Build history of the part. All positions in model axes, mm. A direction names the side the tool comes from. Round coordinates to 2 decimals unless told otherwise and drop trailing zeros. Loops run counter-clockwise (first coordinate to the right, second up) from the corner with the lowest first, then second, coordinate; pieces in that order, holes last. Notation, with made-up numbers: (-34, 4) - (-7, 4) arc R22 cw to (-7, 17) - close; hole circle Ø9 at (-27.5, -17.75). An arc over 180 degrees is marked (long way). Put each result on its own line as item: value. Start each with the question number.
from build123d import *

# Parameters (mm, degrees)
F0_W     = 50.8
F0_H     = 50.8
F1_DEPTH = 7.62
F2_T     = -1.27
F3_W     = 1.27
F3_H     = 6.604
F3_W_2   = 7.62
F3_H_2   = 1.27
F4_DEPTH = 6.35
F5_R     = 1.27
F6_DEPTH = 25.4


with BuildPart() as f1:
    # F0 (on Top) → F1 (new body)
    with BuildSketch(Plane.XY):
        with Locations((25.4, 25.4)):
            Rectangle(F0_W, F0_H)
    extrude(amount=F1_DEPTH)

    # F2
    f2_openings = [f1.faces().sort_by_distance(p)[0] for p in [
        (25.4, 25.4, 7.62),
    ]]
    offset(amount=F2_T, openings=f2_openings)

    # F3 (on face) → F4 (join)
    with BuildSketch(Plane.XY.offset(1.27)):
        Polygon((6.35, 42.545278), (6.35, 1.27), (7.62, 1.27), (7.62, 41.275278), (7.62, 42.545278), align=None)
        Polygon((7.62, 42.545278), (7.62, 41.275278), (39.37, 41.275278), (40.64, 41.275278), (40.64, 42.545278), align=None)
        with Locations((40.005, 37.973278)):
            Rectangle(F3_W, F3_H)
        with Locations((24.184101, 35.050092)):
            Rectangle(F3_W_2, F3_H_2)
    extrude(amount=F4_DEPTH)

    # F5 (on face) → F6 (cut)
    with BuildSketch(Plane.XY.offset(1.27)):
        with Locations((3.990767, 5.742811)):
            Circle(F5_R)
        with Locations((3.796095, 10.80427)):
            Circle(F5_R)
    extrude(amount=-F6_DEPTH, mode=Mode.SUBTRACT)


solid = f1.part
Item 1: Slice it at C-C (y = 38). Give the cut face in (x, z), plus the area to 3 significant figures.
Item 2: Two-plate mould, pull along Y, no slides. Class faces 1 (the flat face through (28, 1.27, 4)), 2 (the flat face through (0, 25, 4)), 3 (the flat face through (25, 0, 4)): pulls with the +Y half, pulls with the -Y half, needs draft (parallel to the pull), parting line crosses it, or undercut.
Item 3: Slice it at D-D (x = 44). Give the cut face in (y, z), plus the area to 3 significant figures.
Item 4: Slice it at A-A (z = 7). Give the cut face in (x, y).
Item 5: Drill centre lines: probe 1 along X at (y, z) = (27, 3); probe 2 along Y at (x, z) = (19, 5.75); probe 3 along X at (y, z) = (38.5, 6.75). Where is each one in solid material? Low to high. Write a range as [from, to].
Item 6: Which spindle directions (+Z, -Z, +X, -X, +Y, -Y) get a long thin tool onto all of the face, cutting with end or side? Do faces 4 (the cylindrical face through (3.521, 9.564, 0.644)), 5 (the flat face through (1.27, 25, 4)). Say none if no direction does.
Item 7: Slice it at B-B (x = 16.5). Give the cut face in (y, z), plus the area to 3 significant figures.
Computed values:
1. outline: (0, 0) - (50.8, 0) - (50.8, 7.62) - (49.53, 7.62) - (49.53, 1.27) - (40.64, 1.27) - (40.64, 7.62) - (39.37, 7.62) - (39.37, 1.27) - (7.62, 1.27) - (7.62, 7.62) - (6.35, 7.62) - (6.35, 1.27) - (1.27, 1.27) - (1.27, 7.62) - (0, 7.62) - close
1. area: 96.8 mm^2
2. face 1: undercut
2. face 2: needs draft
2. face 3: pulls with the -Y half
3. outline: (0, 0) - (50.8, 0) - (50.8, 7.62) - (49.53, 7.62) - (49.53, 1.27) - (1.27, 1.27) - (1.27, 7.62) - (0, 7.62) - close
3. area: 80.6 mm^2
4. outline: (0, 0) - (50.8, 0) - (50.8, 50.8) - (0, 50.8) - close; (20.37, 34.42) - (27.99, 34.42) - (27.99, 35.69) - (20.37, 35.69) - close; hole (1.27, 1.27) - (6.35, 1.27) - (6.35, 42.55) - (40.64, 42.55) - (40.64, 34.67) - (39.37, 34.67) - (39.37, 41.28) - (7.62, 41.28) - (7.62, 1.27) - (49.53, 1.27) - (49.53, 49.53) - (1.27, 49.53) - close
5. probe 1: x = [0, 1.27], [6.35, 7.62], [49.53, 50.8]
5. probe 2: y = [0, 1.27], [41.28, 42.55], [49.53, 50.8]
5. probe 3: x = [0, 1.27], [6.35, 7.62], [39.37, 40.64], [49.53, 50.8]
6. face 4: +Z, -Z
6. face 5: +Z
7. outline: (0, 0) - (50.8, 0) - (50.8, 7.62) - (49.53, 7.62) - (49.53, 1.27) - (42.55, 1.27) - (42.55, 7.62) - (41.28, 7.62) - (41.28, 1.27) - (1.27, 1.27) - (1.27, 7.62) - (0, 7.62) - close
7. area: 88.7 mm^2
